from build123d import *

# Parameters (mm, degrees)
SKETCH1_W           = 88.9
SKETCH1_H           = 1720.85
SKETCH1_W_2         = 815.975
SKETCH1_H_2         = 76.2
SKETCH1_W_3         = 816.102
BOSS_EXTRUDE1_DEPTH = 50.8
SKETCH2_W           = 88.9
SKETCH2_H           = 76.2
BOSS_EXTRUDE2_DEPTH = 101.6
SKETCH11_W          = 76.200000018
SKETCH11_H          = 1210.925919092
BOSS_EXTRUDE6_DEPTH = 12.7
SKETCH12_W          = 88.9
SKETCH12_H          = 1215.673478613
BOSS_EXTRUDE7_DEPTH = 12.7
SKETCH13_W          = 76.2
SKETCH13_H          = 1211.38713944
BOSS_EXTRUDE8_DEPTH = 12.7
BOSS_EXTRUDE9_DEPTH = 12.7


with BuildPart() as part:
    # Sketch1 → Boss-Extrude1 (new body)
    with BuildSketch(Plane(origin=(0, 0, 0), x_dir=(1, 0, 0), z_dir=(0, 1, 0))):
        with Locations((44.45, -860.425)):
            Rectangle(SKETCH1_W, SKETCH1_H)
        with Locations((-407.9875, -860.425)):
            Rectangle(SKETCH1_W_2, SKETCH1_H_2)
        with Locations((496.951, -860.425)):
            Rectangle(SKETCH1_W_3, SKETCH1_H_2)
    extrude(amount=BOSS_EXTRUDE1_DEPTH)



with BuildPart() as body_2:
    # Sketch2 → Boss-Extrude2 (new body)
    with BuildSketch(Plane(origin=(0, 914.4, 0), x_dir=(1, 0, 0), z_dir=(0, 1, 0))):
        with Locations((44.45, -860.425)):
            Rectangle(SKETCH2_W, SKETCH2_H)
    extrude(amount=BOSS_EXTRUDE2_DEPTH)


with BuildPart() as part_1:
    add(part.part)

    add(body_2.part)  # Boss-Extrude6 merges body 2
    # Sketch11 → Boss-Extrude6 (add)
    with BuildSketch(Plane(origin=(515.239820979, 469.832103155, -4.562218888), x_dir=(0.004834466277190451, 0.004408408213341139, 0.9999785967073692), z_dir=(-0.7389010285363795, -0.6737822080618631, 0.006542639158684001))):
        with Locations((865.004917385, 33.212637894)):
            Rectangle(SKETCH11_W, SKETCH11_H)
    extrude(amount=BOSS_EXTRUDE6_DEPTH)

    # Sketch12 → Boss-Extrude7 (add)
    with BuildSketch(Plane(origin=(0, 880.564980502, 958.757073848), x_dir=(-1, 0, 0), z_dir=(0, -0.6764357489630263, -0.7365016480122972))):
        with Locations((-44.45, -518.793435578)):
            Rectangle(SKETCH12_W, SKETCH12_H)
    extrude(amount=BOSS_EXTRUDE7_DEPTH)

    # Sketch13 → Boss-Extrude8 (add)
    with BuildSketch(Plane(origin=(-471.041897908, 429.285012176, 0), x_dir=(0, 0, 1), z_dir=(-0.7391076653302462, 0.6735873061824078, 0))):
        with Locations((860.425, 93.609836957)):
            Rectangle(SKETCH13_W, SKETCH13_H)
    extrude(amount=-BOSS_EXTRUDE8_DEPTH)

    # Sketch14 → Boss-Extrude9 (add)
    with BuildSketch(Plane(origin=(0.320485024, 23.523248222, -25.60821453), x_dir=(-0.9999575295340857, 0.006234703363140706, -0.006787311843563117), z_dir=(0.009216242623115463, 0.6764620710773515, -0.7364198036892085))):
        Polygon((-88.579501445, 37.41171492), (0.316722931, 37.41171492), (0.316722931, 1252.792330393), (-88.579501445, 1252.540281398), align=None)
    extrude(amount=-BOSS_EXTRUDE9_DEPTH)


solid = part_1.part
Could you check a few things on this model? Use its own coordinates, in mm. A direction names the side the tool comes from. Give positions to 0.01 mm unless a question says otherwise; leave off trailing zeros. Order: outer loops, then holes, each group sorted by start corner. A loop starts at its lowest first (then second) coordinate and runs counter-clockwise, first axis right, second up. Notation, with made-up numbers: (11, -10.75) -> (22, -10.75) arc R11 ccw to (22, 3.25) -> close; hole circle Ø4 at (82, 42.5). An arc over 180 degrees is marked (long way). Answer in a Markdown table with one row per item. Add a question column.
Item 1: Imagine slicing it at B-B (z = 1218.5). List the corners of the cut face in (x, y) for me.
Item 2: Please list where these lines run through material, in increasing order: probe 1 along Y at (x, z) = (616, 897); probe 2 along Y at (x, z) = (-431, 874.5); probe 3 along X at (y, z) = (745.5, 894.5).
Item 3: We'd pull the mould along Z, two halves only. Please class faces 3 (the flat face through (40, 0, 856)), 4 (the flat face through (44, 981, 898.525)), 5 (the flat face through (45.07, 495.22, 1295.43)): pulls with the +Z half, pulls with the -Z half, needs draft (parallel to the pull), parting line crosses it, or undercut.
Item 4: I'm going to push flat-ended pins straight in: P1, Ø4, axis at x = 3.5, y = 397.5, coming from the +Z side; P2, Ø25, axis at y = 926, z = 845, coming from the +X side; P3, Ø15, axis at y = 31.5, z = 423.5, coming from the -X side; P4, Ø23, axis at x = 33.5, z = 867, coming from the -Y side. Where does each tip first touch, or does it pass through?
Item 5: Imagine slicing it at A-A (x = -127.5). List the corners of the cut face in (y, z) for me (1 decimal).
Item 6: Imagine slicing it at C-C (y = 100). List the corners of the cut face in (x, z) for me (3 decimals).
Item 7: For faces 1 (the flat face through (44, 25, 1720.85)), 2 (the flat face through (88.9, 25, 417)), which set-ups out of +Z, -Z, +X, -X, +Y, -Y let a thin tool reach every point of the face, with its end or its side?
Result:
| question | item | result |
|---|---|---|
| 1 | outline | (0, 0) -> (88.9, 0) -> (88.9, 50.8) -> (0, 50.8) -> close; (0, 578.98) -> (88.9, 578.98) -> (88.9, 597.76) -> (0, 597.76) -> close |
| 2 | probe 1 | 0 to 50.8, 349.24 to 368.09 |
| 2 | probe 2 | 0 to 50.8, 454.37 to 473.22 |
| 2 | probe 3 | -182.86 to -165.68, 254.64 to 271.83 |
| 3 | face 3 | needs draft |
| 3 | face 4 | pulls with the +Z half |
| 3 | face 5 | undercut |
| 4 | P1 | z = 1404.26 |
| 4 | P2 | x = 118.2 |
| 4 | P3 | x = 0 |
| 4 | P4 | y = 0 |
| 5 | outline | (0, 822.3) -> (50.8, 822.3) -> (50.8, 898.5) -> (0, 898.5) -> close; (787.4, 822.3) -> (806.2, 822.3) -> (806.2, 898.5) -> (787.4, 898.5) -> close |
| 6 | outline | (-771.136, 822.325) -> (-753.954, 822.325) -> (-753.954, 898.525) -> (-771.136, 898.525) -> close; (-0.113, 61.882) -> (0.004, 44.638) -> (88.896, 45.75) -> (88.779, 62.995) -> close; (0, 1658.419) -> (88.9, 1658.419) -> (88.9, 1675.663) -> (0, 1675.663) -> close; (842.614, 822.408) -> (859.801, 822.325) -> (860.475, 898.523) -> (843.288, 898.606) -> close |
| 7 | face 1 | +Z, +X, -X, +Y, -Y |
| 7 | face 2 | -Z, +X, +Y, -Y |
